```python
from build123d import *

# Parameters (mm, degrees)
SKETCH1_W      = 7.96
SKETCH1_H      = 7.96
EXTRUDE1_DEPTH = 9.54
SKETCH2_R      = 2.425
EXTRUDE2_DEPTH = 1.8
SHELL1_T       = -1.55
SKETCH3_W      = 4.86
SKETCH3_H      = 4.86
EXTRUDE3_DEPTH = 0.14
SKETCH5_W      = 1.555
SKETCH5_H      = 7.96
EXTRUDE5_DEPTH = 7.94
SKETCH7_W      = 0.7
SKETCH7_H      = 4.86
EXTRUDE6_DEPTH = 6.53
EXTRUDE7_REACH = 9.96
SKETCH4_W      = 4.86
SKETCH4_H      = 4.86
SKETCH8_R      = 2.425
EXTRUDE8_DEPTH = 1.555
SKETCH9_R      = 1.565
EXTRUDE9_DEPTH = 8.96


with BuildPart() as part:
    # Sketch1 → Extrude1 (new body)
    with BuildSketch(Plane(origin=(0, 0, 0), x_dir=(1, 0, 0), z_dir=(0, 1, 0))):
        Rectangle(SKETCH1_W, SKETCH1_H)
    extrude(amount=EXTRUDE1_DEPTH)

    # Sketch2 → Extrude2 (add)
    with BuildSketch(Plane(origin=(0, 9.54, 0), x_dir=(1, 0, 0), z_dir=(0, 1, 0))):
        Circle(SKETCH2_R)
    extrude(amount=EXTRUDE2_DEPTH)

    # Shell1
    shell1_openings = [part.faces().sort_by_distance(p)[0] for p in [
        (0, 0, 0),
    ]]
    offset(amount=SHELL1_T, openings=shell1_openings, kind=Kind.INTERSECTION)

    # Sketch3 → Extrude3 (cut)
    with BuildSketch(Plane.XZ.offset(-7.99)):
        Rectangle(SKETCH3_W, SKETCH3_H)
    extrude(amount=-EXTRUDE3_DEPTH, mode=Mode.SUBTRACT)

    # Sketch5 → Extrude5 (cut)
    with BuildSketch(Plane(origin=(0, 9.54, 0), x_dir=(1, 0, 0), z_dir=(0, 1, 0))):
        with Locations((-3.2025, 0)):
            Rectangle(SKETCH5_W, SKETCH5_H)
    extrude(amount=-EXTRUDE5_DEPTH, mode=Mode.SUBTRACT)

    # Sketch7 → Extrude6 (add)
    with BuildSketch(Plane.XZ.offset(-8.13)):
        with Locations((-2.075, 0)):
            Rectangle(SKETCH7_W, SKETCH7_H)
        with Locations((2.08, 0)):
            Rectangle(SKETCH7_W, SKETCH7_H)
    extrude(amount=EXTRUDE6_DEPTH)

    # Sketch4 → Extrude7 (cut, up to next)
    with BuildSketch(Plane(origin=(3.98, 0, 0), x_dir=(0, 0, -1), z_dir=(1, 0, 0)), mode=Mode.PRIVATE) as extrude7_sk1:
        with Locations((0, 5.56)):
            Rectangle(SKETCH4_W, SKETCH4_H)
    extrude7_tool1 = extrude(extrude7_sk1.sketch, amount=-EXTRUDE7_REACH, mode=Mode.PRIVATE) & part.part
    add(extrude7_tool1.solids().sort_by_distance((3.98, 5.56, 0))[0], mode=Mode.SUBTRACT)

    # Sketch8 → Extrude8 (add)
    with BuildSketch(Plane.ZY.offset(2.425)):
        with Locations((0, 5.56)):
            Circle(SKETCH8_R)
    extrude(amount=EXTRUDE8_DEPTH)

    # Sketch9 → Extrude9 (cut, through all)
    with BuildSketch(Plane.ZY.offset(3.98)):
        with Locations((0, 5.56)):
            Circle(SKETCH9_R)
    extrude(amount=-EXTRUDE9_DEPTH, mode=Mode.SUBTRACT)


solid = part.part
```
Source: CAD feature listing. Evaluate the final solid. Frame: model axes, mm. A direction names the side the tool comes from. Coordinates: 2 decimals unless noted, no trailing zeros. Write each loop counter-clockwise with the first axis right and the second up, starting at its lowest first coordinate (ties: lowest second). Pieces come first, ordered by that corner, then holes. Notation, with made-up numbers: (42, 56.5) - (99, 56.5) arc R15 ccw to (99, 63.5) - close; hole circle Ø11 at (81, 35.25). An arc over 180 degrees is marked (long way). Answer as a JSON object with one key per item and string values.
Q1. Section query D-D, the plane x = 0. Output: boundary loops of the cut face in (y, z) (3 decimals).
Ans:
{"outline": "(0, -3.98) - (9.54, -3.98) - (9.54, -2.425) - (11.34, -2.425) - (11.34, 2.425) - (9.54, 2.425) - (9.54, 3.98) - (0, 3.98) - (0, 2.43) - (8.13, 2.43) - (8.13, 0.875) - (9.79, 0.875) - (9.79, -0.875) - (8.13, -0.875) - (8.13, -2.43) - (0, -2.43) - close"}
Q2. First-contact query: pin 1 Ø1.9 at (x, z) = (-0.5, 0) entering from -Y; pin 2 Ø0.8 at (y, z) = (2.5, -1) entering from -X (3 decimals). Flat tips, straight axial feed; report the tip coordinate or a pass-through.
Ans:
{"pin 1": "stops at y = 8.13", "pin 2": "stops at x = -2.425"}
Q3. Section query A-A, the plane y = 5.56. Output: boundary loops of the cut face in (x, z) (3 decimals).
Ans:
{"outline": "(-3.98, -2.425) - (-2.425, -2.425) - (-2.425, -3.98) - (3.98, -3.98) - (3.98, -2.43) - (-1.725, -2.43) - (-1.725, -1.565) - (-3.98, -1.565) - close; (-3.98, 1.565) - (-1.725, 1.565) - (-1.725, 2.43) - (3.98, 2.43) - (3.98, 3.98) - (-2.425, 3.98) - (-2.425, 2.425) - (-3.98, 2.425) - close"}
Q4. Section query B-B, the plane x = -2.75. Output: boundary loops of the cut face in (y, z) (3 decimals), plus the area to 3 significant figures.
Ans:
{"outline": "(0, -3.98) - (1.6, -3.98) - (1.6, 3.98) - (0, 3.98) - close; circle Ø4.85 at (5.56, 0); hole circle Ø3.13 at (5.56, 0)", "area": "23.5 mm2"}
Q5. Material intervals for line 1 (Y direction, x = -2.8, z = 0) (3 decimals); line 2 (Z direction, x = 0.75, y = 1.75); line 3 (Z direction, x = 0, y = 8.65) (3 decimals), sorted ascending. Write a range as [from, to].
Ans:
{"line 1": "y = [0, 1.6], [3.135, 3.995], [7.125, 7.985]", "line 2": "z = [-3.98, -2.43], [2.43, 3.98]", "line 3": "z = [-3.98, -0.875], [0.875, 3.98]"}
Q6. Section query C-C, the plane z = 2. Output: boundary loops of the cut face in (x, y) (3 decimals).
Ans:
{"outline": "(-3.98, 0) - (-2.43, 0) - (-2.43, 1.6) - (-3.98, 1.6) - close; (-3.98, 4.189) - (-2.425, 4.189) - (-2.425, 1.6) - (-1.725, 1.6) - (-1.725, 8.13) - (1.73, 8.13) - (1.73, 7.99) - (3.98, 7.99) - (3.98, 9.54) - (1.371, 9.54) - (1.371, 11.34) - (-1.371, 11.34) - (-1.371, 9.54) - (-2.425, 9.54) - (-2.425, 6.931) - (-3.98, 6.931) - close; (1.73, 1.6) - (2.43, 1.6) - (2.43, 0) - (3.98, 0) - (3.98, 3.13) - (1.73, 3.13) - close"}
Q7. Set-up query: faces 5 (the cylindrical face through (-3.192, 7.605, 1.304)), 6 (the flat face through (3, 3.13, 0)), 7 (the flat face through (1, 8.13, 1)), 8 (the cylindrical face through (2.313, 10.427, -0.728)), 9 (the flat face through (1, 4, 2.43)). Return all of +Z, -Z, +X, -X, +Y, -Y with unobstructed straight access to the full face (end or side cutting, diameter ignored); none if empty.
Ans:
{"face 5": "-X", "face 6": "+X", "face 7": "-Y", "face 8": "+Y", "face 9": "none"}
Q8. Draft query along Y for faces 1 (the flat face through (0, 0, -3)), 2 (the cylindrical face through (-0.694, 8.948, 0.532)), 3 (the flat face through (-3, 1.6, 0)), 4 (the flat face through (0, 11.34, 0)). Return one class per face: released by +Y, released by -Y, zero draft, split by the parting line, or undercut.
Ans:
{"face 1": "released by -Y", "face 2": "zero draft", "face 3": "undercut", "face 4": "released by +Y"}
